The listing builds one solid part. Answer for the finished solid, in the listing's coordinates (mm). Face numbers are marked on the shaded views. A direction names the side the tool comes from. Round coordinates to 2 decimals unless told otherwise and drop trailing zeros. Write each loop counter-clockwise with the first axis right and the second up, starting at its lowest first coordinate (ties: lowest second). Pieces come first, ordered by that corner, then holes. Notation, with made-up numbers: (50.5, 33) - (108.5, 33) arc R10 cw to (108.5, 37) - close; hole circle Ø4 at (43.25, -18.5). An arc over 180 degrees is marked (long way). Return JSON: item names as keys, results as strings. Group by question number.
(1) Each of these flat-tipped pins is pushed along its axis until it touches: pin 1 (3.5 mm diameter, centred on x = 64.11, y = 32.46, fed in from +Z); pin 2 (5 mm diameter, centred on x = 16.5, z = 12.5, fed in from +Y); pin 3 (12 mm diameter, centred on x = 22.5, y = 6.5, fed in from -Z); pin 4 (4 mm diameter, centred on y = -16, z = 22.5, fed in from -X). Where does it stop, or does it pass through?
(2) Which of the six approach directions +Z, -Z, +X, -X, +Y, -Y give full straight-line access (tool end or side, diameter ignored) to the marked faces 1, 2 and 3?
(3) Section B-B, the plane z = 16 is taken. Write down the section's boundary in (x, y).
(4) Section C-C, the plane x = 17.5 is taken. Write down the section's boundary in (y, z), then the cut area to 3 significant figures.
(5) Determine the mould class of the marked faces 4, 5, 6 and 7 for opening direction Z: +Z half, -Z half, draft (parallel to the pull), parting line (faces both ways), or undercut.
(6) Find the intervals of material crossed by line 1 along Y through (x, z) = (-9, 21.5); line 2 along Z through (x, y) = (-13, 39.5); line 3 along X through (y, z) = (33.5, 16.5), in increasing order. Write a range as [from, to].
(7) Section A-A, the plane y = 42 is taken. Write down the section's boundary in (x, z).
(8) Section D-D, the plane y = -25 is taken. Write down the section's boundary in (x, z).
```python
from build123d import *

# Parameters (mm, degrees)
F0_R     = 2
F1_DEPTH = 33
F2_W     = 54
F2_H     = 29
F3_DEPTH = 15


with BuildPart() as f1:
    # F0 (on Top) → F1 (new body)
    with BuildSketch(Plane.XY):
        with BuildLine():
            Line((38.111041, 50.456811), (-19.888959, 50.456811))
            Line((-19.888959, 50.456811), (-19.888959, -3.543189))
            ThreePointArc((-19.888959, -3.543189), (-16.820127, -19.241913), (-8.065448, -32.629344))
            Line((-8.065448, -32.629344), (-11.31872, -35.904956))
            Line((-11.31872, -35.904956), (-11.550578, -36.138406))
            ThreePointArc((-11.550578, -36.138406), (-11.238961, -43.254993), (-4.12779, -42.83767))
            Line((-4.12779, -42.83767), (-0.589658, -38.798335))
            ThreePointArc((-0.589658, -38.798335), (57.368005, -33.227692), (63.697868, 24.651973))
            Line((63.697868, 24.651973), (67.779562, 29.059465))
            ThreePointArc((67.779562, 29.059465), (67.475048, 36.155927), (60.381633, 35.787204))
            Line((60.381633, 35.787204), (56.727759, 32.172584))
            ThreePointArc((56.727759, 32.172584), (47.901206, 37.046076), (38.111041, 39.456811))
            Line((38.111041, 39.456811), (38.111041, 50.456811))
        make_face()
        with Locations((-7.888959, -39.543189)):
            Circle(F0_R, mode=Mode.SUBTRACT)
        with BuildLine():
            ThreePointArc((-5.091348, -35.399112), (-4.707802, -35.685698), (-4.353425, -36.007655))
            ThreePointArc((-4.353425, -36.007655), (-4.724132, -35.7055), (-5.091348, -35.399112))
        make_face(mode=Mode.SUBTRACT)
        with Locations((64.111041, 32.456811)):
            Circle(F0_R, mode=Mode.SUBTRACT)
    extrude(amount=F1_DEPTH)

    # F2 (on face) → F3 (cut)
    with BuildSketch(Plane(origin=(0, 50.456811, 0), x_dir=(-1, 0, 0), z_dir=(0, 1, 0))):
        with Locations((-9.111041, 16.5)):
            Rectangle(F2_W, F2_H)
    extrude(amount=-F3_DEPTH, mode=Mode.SUBTRACT)


solid = f1.part
```
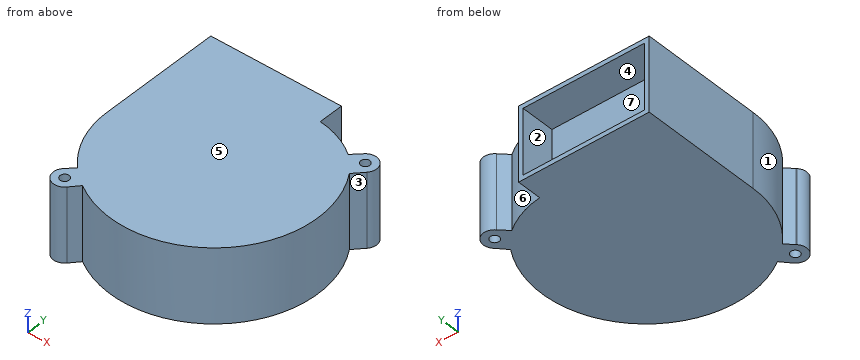
Working result:
{
 "1": {"pin 1": "passes through", "pin 2": "stops at y = 35.46", "pin 3": "stops at z = 0", "pin 4": "stops at x = -18.56"},
 "2": {"face 1": "+Z, -Z, -X", "face 2": "+Y", "face 3": "+Z, -Z, +X"},
 "3": {"outline": "(-19.89, -3.54) arc R41.69 ccw to (-8.07, -32.63) - (-11.32, -35.9) - (-11.55, -36.14) arc R5 ccw (long way) to (-4.13, -42.84) - (-0.59, -38.8) arc R46.13 ccw to (63.7, 24.65) - (67.78, 29.06) arc R5 ccw (long way) to (60.38, 35.79) - (56.73, 32.17) arc R38.44 ccw to (38.11, 39.46) - (38.11, 50.46) - (36.11, 50.46) - (36.11, 35.46) - (-17.89, 35.46) - (-17.89, 50.46) - (-19.89, 50.46) - close; hole circle Ø4 at (-7.89, -39.54); hole (-5.09, -35.4) arc R41.69 ccw to (-4.35, -36.01) arc R5 ccw to start; hole circle Ø4 at (64.11, 32.46)"},
 "4": {"outline": "(-45.92, 0) - (50.46, 0) - (50.46, 2) - (35.46, 2) - (35.46, 31) - (50.46, 31) - (50.46, 33) - (-45.92, 33) - close", "area": "2,750 mm^2"},
 "5": {"face 4": "undercut", "face 5": "+Z half", "face 6": "draft", "face 7": "undercut"},
 "6": {"line 1": "y = [-44.42, -41.21], [-37.88, -33.57], [-31.64, 35.46]", "line 2": "z = [0, 2], [31, 33]", "line 3": "x = [-19.89, 54.81], [58.07, 62.4], [65.82, 69]"},
 "7": {"outline": "(-19.89, 0) - (38.11, 0) - (38.11, 33) - (-19.89, 33) - close; hole (-17.89, 2) - (36.11, 2) - (36.11, 31) - (-17.89, 31) - close"},
 "8": {"outline": "(-13.94, 0) - (63.98, 0) - (63.98, 33) - (-13.94, 33) - close"}
}
